Could you check a few things on this model? Use its own coordinates, in mm. Round coordinates to 2 decimals unless told otherwise and drop trailing zeros. Write each loop counter-clockwise with the first axis right and the second up, starting at its lowest first coordinate (ties: lowest second). Pieces come first, ordered by that corner, then holes.
```python
from build123d import *

# Parameters (mm, degrees)
SKETCH1_R           = 36.3093
BOSS_EXTRUDE1_DEPTH = 3.175
CUT_EXTRUDE1_DEPTH  = 52.44716861
SKETCH3_R           = 1.505
SKETCH3_R_2         = 2.54
CUT_EXTRUDE2_DEPTH  = 52.44716861


with BuildPart() as part:
    # Sketch1 → Boss-Extrude1 (new body)
    with BuildSketch(Plane.XY):
        Circle(SKETCH1_R)
    extrude(amount=BOSS_EXTRUDE1_DEPTH)

    # Sketch2 → Cut-Extrude1 (cut, through all)
    with BuildSketch(Plane.XY.offset(3.175)):
        with BuildLine():
            Line((-24.593444248, -6.35), (-7.931147458, -6.35))
            ThreePointArc((-7.931147458, -6.35), (0, -10.16), (7.931147458, -6.35))
            Line((7.931147458, -6.35), (24.593444248, -6.35))
            ThreePointArc((24.593444248, -6.35), (0, -25.4), (-24.593444248, -6.35))
        make_face()
        with BuildLine():
            Line((7.931147458, 6.35), (24.593444248, 6.35))
            ThreePointArc((24.593444248, 6.35), (0, 25.4), (-24.593444248, 6.35))
            Line((-24.593444248, 6.35), (-7.931147458, 6.35))
            ThreePointArc((-7.931147458, 6.35), (0, 10.16), (7.931147458, 6.35))
        make_face()
    extrude(amount=-CUT_EXTRUDE1_DEPTH, mode=Mode.SUBTRACT)

    # Sketch3 → Cut-Extrude2 (cut, through all)
    with BuildSketch(Plane.XY.offset(3.175)):
        with Locations((-4.699, 0)):
            Circle(SKETCH3_R)
        with Locations((4.699, 0)):
            Circle(SKETCH3_R)
        Circle(SKETCH3_R_2)
    extrude(amount=-CUT_EXTRUDE2_DEPTH, mode=Mode.SUBTRACT)


solid = part.part
```
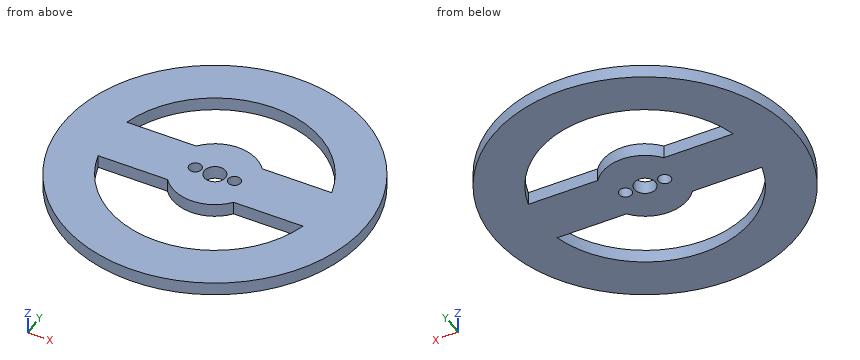
Q1. Imagine slicing it at C-C, the plane y = 0. Write out the boundary of the cut face in (x, z) (3 decimals).
Q2. Imagine slicing it at D-D, the plane x = 15. Write out the boundary of the cut face in (y, z) (3 decimals), then the cut area to 3 significant figures.
Q3. I'm going to push flat-ended pins straight in: pin 1 Ø4 at (x, y) = (-15.5, -20) entering from -Z; pin 2 Ø1.5 at (x, z) = (24.5, 2.5) entering from -Y; pin 3 Ø1.5 at (x, z) = (-4.5, 0.5) entering from +Y; pin 4 Ø1 at (x, z) = (15, 2) entering from -Y. Where does each tip first touch, or does it pass through?
Q4. If I drill on L1, parallel to Y at x = 0, z = 1.35; L2, parallel to Y at x = 17, z = 2.4; L3, parallel to Y at x = 18.5, z = 1.8, over which ranges is the centre line in solid material (lowest first)?
Q5. Imagine slicing it at B-B, the plane x = 0. Write out the boundary of the cut face in (y, z) (3 decimals).
Q6. Imagine slicing it at A-A, the plane z = 1.4. Write out the boundary of the cut face in (x, y) (3 decimals).
Results found:
1. outline: (-36.309, 0) - (-6.204, 0) - (-6.204, 3.175) - (-36.309, 3.175) - close; (-3.194, 0) - (-2.54, 0) - (-2.54, 3.175) - (-3.194, 3.175) - close; (2.54, 0) - (3.194, 0) - (3.194, 3.175) - (2.54, 3.175) - close; (6.204, 0) - (36.309, 0) - (36.309, 3.175) - (6.204, 3.175) - close
2. outline: (-33.066, 0) - (-20.498, 0) - (-20.498, 3.175) - (-33.066, 3.175) - close; (-6.35, 0) - (6.35, 0) - (6.35, 3.175) - (-6.35, 3.175) - close; (20.498, 0) - (33.066, 0) - (33.066, 3.175) - (20.498, 3.175) - close
2. area: 120 mm2
3. pin 1: stops at z = 0
3. pin 2: stops at y = -27.46
3. pin 3: stops at y = 36.12
3. pin 4: stops at y = -33.29
4. L1: y = -36.31 to -25.4, -10.16 to -2.54, 2.54 to 10.16, 25.4 to 36.31
4. L2: y = -32.08 to -18.87, -6.35 to 6.35, 18.87 to 32.08
4. L3: y = -31.24 to -17.4, -6.35 to 6.35, 17.4 to 31.24
5. outline: (-36.309, 0) - (-25.4, 0) - (-25.4, 3.175) - (-36.309, 3.175) - close; (-10.16, 0) - (-2.54, 0) - (-2.54, 3.175) - (-10.16, 3.175) - close; (2.54, 0) - (10.16, 0) - (10.16, 3.175) - (2.54, 3.175) - close; (25.4, 0) - (36.309, 0) - (36.309, 3.175) - (25.4, 3.175) - close
6. outline: circle Ø72.619 at (0, 0); hole (-24.593, -6.35) arc R25.4 ccw to (24.593, -6.35) - (7.931, -6.35) arc R10.16 cw to (-7.931, -6.35) - close; hole (-24.593, 6.35) - (-7.931, 6.35) arc R10.16 cw to (7.931, 6.35) - (24.593, 6.35) arc R25.4 ccw to start; hole circle Ø3.01 at (-4.699, 0); hole circle Ø5.08 at (0, 0); hole circle Ø3.01 at (4.699, 0)
